Verification items for the finished model (mm, model axes). Face numbers are marked on the shaded views. A direction names the side the tool comes from. Round coordinates to 2 decimals unless told otherwise and drop trailing zeros. Order: outer loops, then holes, each group sorted by start corner. A loop starts at its lowest first (then second) coordinate and runs counter-clockwise, first axis right, second up. Notation, with made-up numbers: (68.5, 35.25) -> (99.5, 35.25) arc R19 ccw to (99.5, 60.25) -> close; hole circle Ø7 at (-14, 0). An arc over 180 degrees is marked (long way). Write item = value, one per line. Start each with the question number.
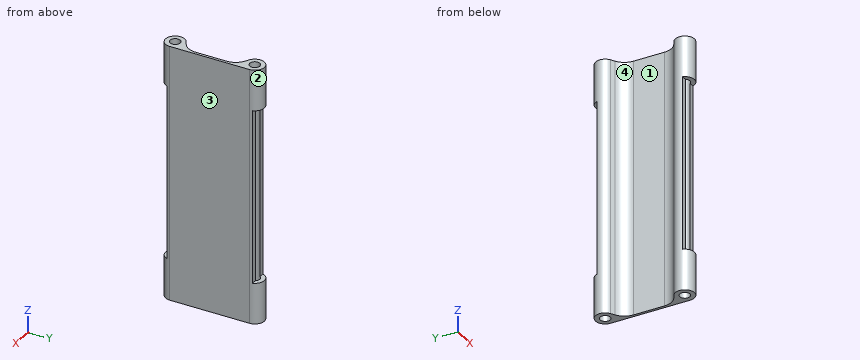
from build123d import *

# Parameters (mm, degrees)
CROQUIS1_R              = 3.175
SALIENTE_EXTRUIR1_DEPTH = 160
REDONDEO1_R             = 10
CROQUIS3_W              = 108.791812306
CROQUIS3_H              = 18.145434914
CORTAR_EXTRUIR2_DEPTH   = 13


with BuildPart() as part:
    # Croquis1 → Saliente-Extruir1 (new body)
    with BuildSketch(Plane.XY):
        with BuildLine():
            Line((-1.6, 15.556228096), (-8.98691391, 19.796314259))
            ThreePointArc((-8.98691391, 19.796314259), (-9.006535925, 30.19237342), (0, 25))
            Line((0, 25), (0, -25))
            ThreePointArc((0, -25), (-9.006535925, -30.19237342), (-8.98691391, -19.796314259))
            Line((-8.98691391, -19.796314259), (-1.6, -15.556228096))
            Line((-1.6, -15.556228096), (-1.6, 15.556228096))
        make_face()
        with Locations((-6, 25)):
            Circle(CROQUIS1_R, mode=Mode.SUBTRACT)
        with Locations((-6, -25)):
            Circle(CROQUIS1_R, mode=Mode.SUBTRACT)
    extrude(amount=-SALIENTE_EXTRUIR1_DEPTH)

    # Redondeo1
    redondeo1_edges = [part.edges().sort_by_distance(p)[0] for p in [
        (-1.6, -15.556228096, -80),
        (-1.6, 15.556228096, -80),
    ]]
    fillet(redondeo1_edges, radius=REDONDEO1_R)

    # Croquis3 → Cortar-Extruir2 (cut, through all)
    with BuildSketch(Plane(origin=(0, 0, 0), x_dir=(0, 0, -1), z_dir=(1, 0, 0))):
        with Locations((80, 35.875128035)):
            Rectangle(CROQUIS3_W, CROQUIS3_H)
        with Locations((80, -35.875128035)):
            Rectangle(CROQUIS3_W, CROQUIS3_H)
    extrude(amount=-CORTAR_EXTRUIR2_DEPTH, mode=Mode.SUBTRACT)


solid = part.part
(1) Set-up check for the marked faces 1 and 2: record each of +Z, -Z, +X, -X, +Y, -Y from which the full face is reachable in a straight line by a thin tool's end or side.
(2) Cross-section at B-B (z = -106.5). Enter the section's corners in (x, y) (3 decimals).
(3) Scan lines: line 1 along Z through (x, y) = (-2.5, 28.5); line 2 along Y through (x, z) = (-6, -62.5) (3 decimals); line 3 along X through (y, z) = (9, -125.5). Record each from-to range of solid material in increasing order. Write a range as from..to.
(4) Cross-section at D-D (y = -17). Enter the section's corners in (x, z), and give its area (3 significant figures).
(5) Draft check along Y on the marked faces 3 and 4. Enter one of: +Y half, -Y half, draft (parallel to the pull), parting line (faces both ways), or undercut.
(6) Depth check by flat-ended pin: pin 1 (0.9 mm diameter, centred on x = -10, z = -95.5, fed in from -Y); pin 2 (3 mm diameter, centred on y = -12, z = -132, fed in from -X); pin 3 (3 mm diameter, centred on x = -5.5, z = -61, fed in from +Y); pin 4 (2 mm diameter, centred on x = -8.5, y = 28, fed in from +Z). Enter the tip coordinate at first touch or a pass-through.
(7) Cross-section at A-A (z = -14.5). Enter the section's corners in (x, y) (3 decimals).
(8) Cross-section at C-C (y = 1). Enter the section's corners in (x, z).
Outcome:
q1.face_1 = +Z, -Z, -X
q1.face_2 = +Z, -Z
q2.outline = (-11.723, -26.802) -> (-8.614, -26.802) arc R3.175 cw (long way) to (-3.386, -26.802) -> (-0.277, -26.802) arc R6 ccw to (0, -25) -> (0, 25) arc R6 ccw to (-0.277, 26.802) -> (-3.386, 26.802) arc R3.175 cw (long way) to (-8.614, 26.802) -> (-11.723, 26.802) arc R6 ccw to (-8.987, 19.796) -> (-6.622, 18.439) arc R10 cw to (-1.6, 9.766) -> (-1.6, -9.766) arc R10 cw to (-6.622, -18.439) -> (-8.987, -19.796) arc R6 ccw to start
q3.line_1 = -160..-134.4, -25.6..0
q3.line_2 = -21.825..-18.051, 18.051..21.825
q3.line_3 = -1.6..0
q4.outline = (-4.7, -160) -> (0, -160) -> (0, 0) -> (-4.7, 0) -> close
q4.area = 751 mm^2
q5.face_3 = draft
q5.face_4 = undercut
q6.pin_1 = -26.8
q6.pin_2 = -2.32
q6.pin_3 = 22.53
q6.pin_4 = 0
q7.outline = (-8.987, -19.796) arc R6 ccw (long way) to (0, -25) -> (0, 25) arc R6 ccw (long way) to (-8.987, 19.796) -> (-6.622, 18.439) arc R10 cw to (-1.6, 9.766) -> (-1.6, -9.766) arc R10 cw to (-6.622, -18.439) -> close; hole circle Ø6.35 at (-6, -25); hole circle Ø6.35 at (-6, 25)
q8.outline = (-1.6, -160) -> (0, -160) -> (0, 0) -> (-1.6, 0) -> close
